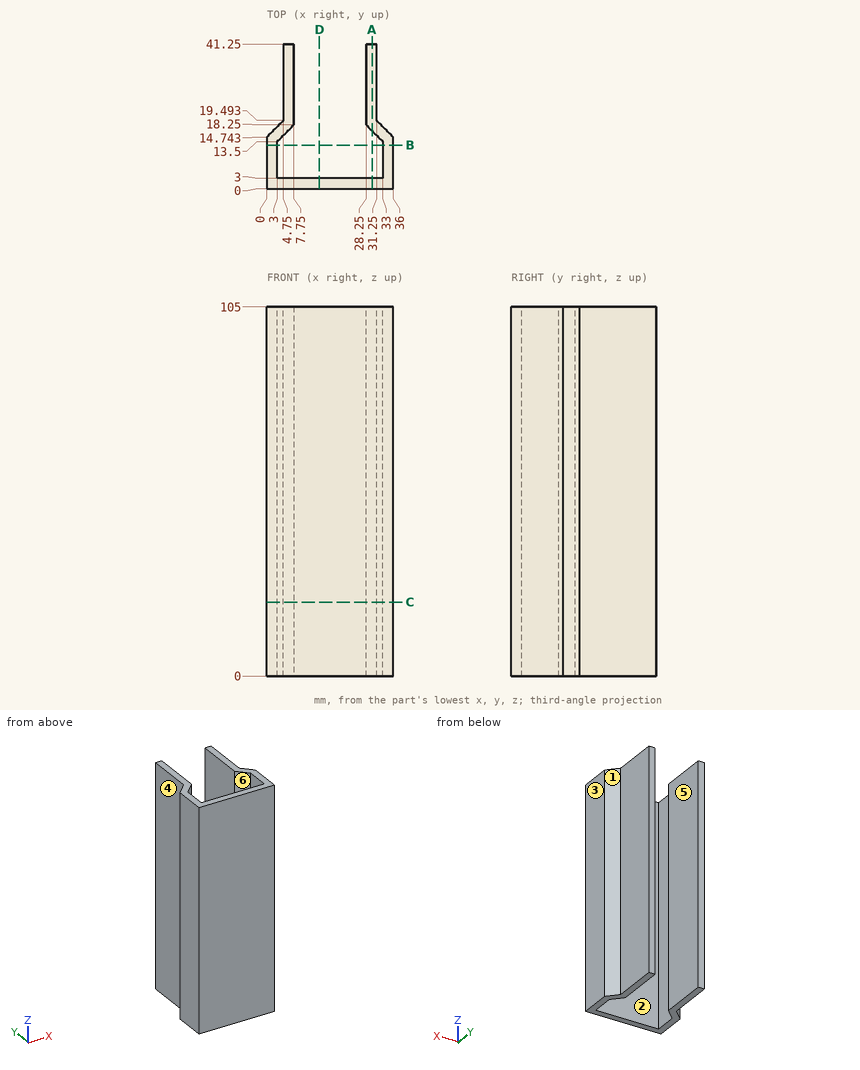
Source: three-view drawing plus pictorial views. Frame: mm from the lowest corner of the part. A direction names the side the tool comes from. Round coordinates to 2 decimals unless told otherwise and drop trailing zeros. Loops run counter-clockwise (first coordinate to the right, second up) from the corner with the lowest first, then second, coordinate; pieces in that order, holes last. Notation, with made-up numbers: (24, -24) - (65, -24) arc R15 cw to (65, -16) - close; hole circle Ø6 at (38.25, -11). An arc over 180 degrees is marked (long way). Write each question's results on one line, items separated by ' | '. Start each with the question number.
1) First-contact query: P1, Ø10, axis at x = 12, y = 23.5, coming from the +Z side; P2, Ø7, axis at y = 27.5, z = 54, coming from the +X side; P3, Ø1.5, axis at y = 31, z = 41.5, coming from the -X side. Flat tips, straight axial feed; report the tip coordinate or a pass-through.
2) Access query for the marked faces 4, 5 and 6. Directions: +Z, -Z, +X, -X, +Y, -Y. A direction counts if a zero-diameter tool reaches every point of the face in a straight line with its end or side. Return the directions, or none.
3) Cut plane C-C on z = 21. Return loops of the section in (x, y), then the cut area to 3 significant figures.
4) Cut plane D-D on x = 15. Return loops of the section in (y, z).
5) Cut plane A-A on x = 30. Return loops of the section in (y, z), then the cut area to 3 significant figures.
6) Mould query, pull axis Y, two halves, no side actions, for the marked faces 1, 2 and 3. Classes: released by +Y, released by -Y, zero draft, split by the parting line, or undercut.
7) Line query: probe 1 along X at (y, z) = (36, 11.5); probe 2 along X at (y, z) = (11.5, 15); probe 3 along Y at (x, z) = (15, 52.5). Output: solid intervals per line, ascending. Write a range as [from, to].
8) Cut plane B-B on y = 12.5. Return loops of the section in (x, z).
Verdict:
1) P1: stops at z = 105 | P2: stops at x = 31.25 | P3: stops at x = 4.75
2) face 4: +Z, -Z, -X, +Y | face 5: +Z, -Z, +Y | face 6: +Z, -Z
3) outline: (0, 0) - (36, 0) - (36, 14.74) - (31.25, 19.49) - (31.25, 41.25) - (28.25, 41.25) - (28.25, 18.25) - (33, 13.5) - (33, 3) - (3, 3) - (3, 13.5) - (7.75, 18.25) - (7.75, 41.25) - (4.75, 41.25) - (4.75, 19.49) - (0, 14.74) - close | area: 349 mm2
4) outline: (0, 0) - (3, 0) - (3, 105) - (0, 105) - close
5) outline: (0, 0) - (3, 0) - (3, 105) - (0, 105) - close; (16.5, 0) - (41.25, 0) - (41.25, 105) - (16.5, 105) - close | area: 2,910 mm2
6) face 1: released by +Y | face 2: undercut | face 3: zero draft
7) probe 1: x = [4.75, 7.75], [28.25, 31.25] | probe 2: x = [0, 3], [33, 36] | probe 3: y = [0, 3]
8) outline: (0, 0) - (3, 0) - (3, 105) - (0, 105) - close; (33, 0) - (36, 0) - (36, 105) - (33, 105) - close
